Print and shaded views of the part. All mm, measured from the part's lowest x, y and z. A direction names the side the tool comes from. Give positions to 0.01 mm unless a question says otherwise; leave off trailing zeros. Order: outer loops, then holes, each group sorted by start corner. A loop starts at its lowest first (then second) coordinate and runs counter-clockwise, first axis right, second up. Notation, with made-up numbers: (-39, -15) - (-25, -15) arc R30 ccw to (-25, 16) - close; hole circle Ø5 at (25.25, 70). An arc over 180 degrees is marked (long way). Answer in a Markdown table with one row per item.
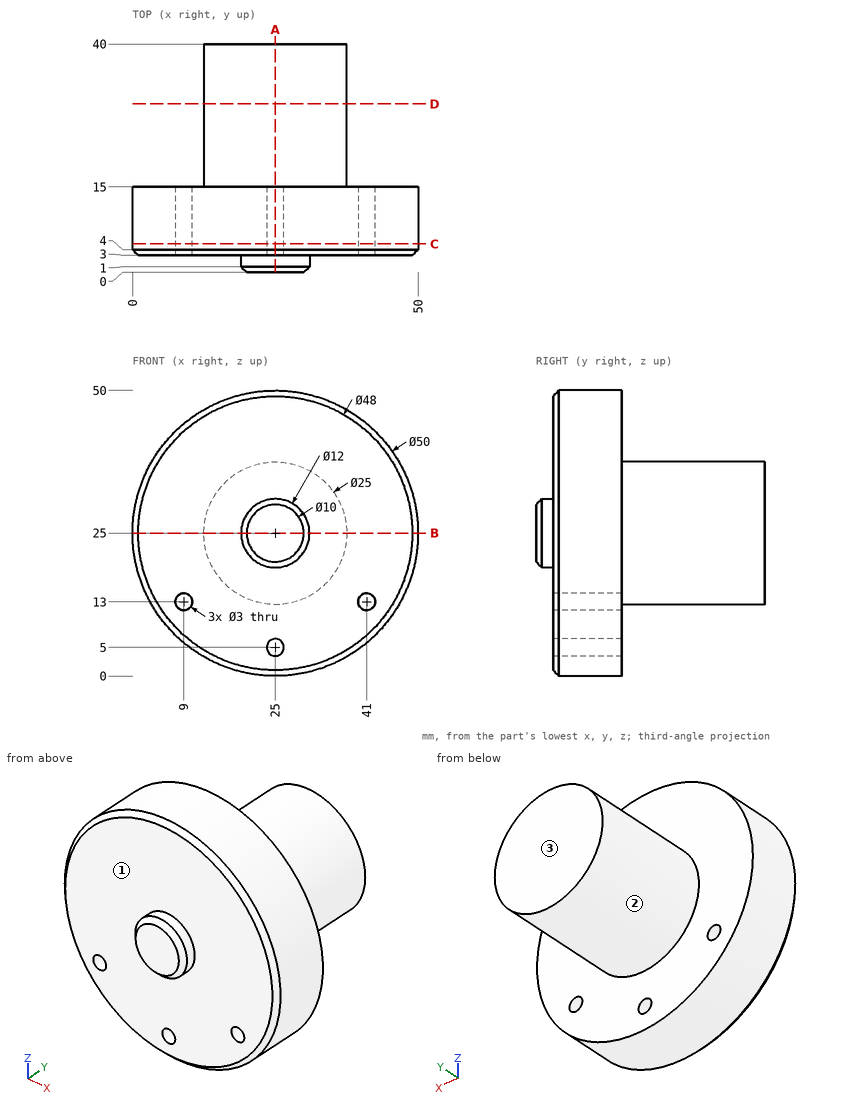
1. Cut at B-B on z = 25. Write the cut outline in (x, y).
Check result:
| item | result |
|---|---|
| outline | (0, 4) - (1, 3) - (19, 3) - (19, 1) - (20, 0) - (30, 0) - (31, 1) - (31, 3) - (49, 3) - (50, 4) - (50, 15) - (37.5, 15) - (37.5, 40) - (12.5, 40) - (12.5, 15) - (0, 15) - close |
2. Cut at D-D on y = 29.5. Write the cut outline in (x, z), and give its area (3 significant figures).
Check result:
| item | result |
|---|---|
| outline | circle Ø25 at (25, 25) |
| area | 491 mm² |
3. Probe line 1 (X direction, y = 9.5, z = 13); line 2 (Y direction, x = 40, z = 16.5); line 3 (Y direction, x = 15, z = 18.5). List the from-to ranges inside material, lowest first.
Check result:
| item | result |
|---|---|
| line 1 | x = 3.07 to 7.5, 10.5 to 39.5, 42.5 to 46.93 |
| line 2 | y = 3 to 15 |
| line 3 | y = 3 to 40 |
4. Cut at C-C on y = 5. Write the cut outline in (x, z), and give its area (3 significant figures).
Check result:
| item | result |
|---|---|
| outline | circle Ø50 at (25, 25); hole circle Ø3 at (9, 13); hole circle Ø3 at (25, 5); hole circle Ø3 at (41, 13) |
| area | 1,940 mm² |
5. Cut at A-A on x = 25. Write the cut outline in (y, z), and give its area (3 significant figures).
Check result:
| item | result |
|---|---|
| outline | (0, 20) - (1, 19) - (3, 19) - (3, 6.5) - (15, 6.5) - (15, 12.5) - (40, 12.5) - (40, 37.5) - (15, 37.5) - (15, 50) - (4, 50) - (3, 49) - (3, 31) - (1, 31) - (0, 30) - close; (3, 1) - (4, 0) - (15, 0) - (15, 3.5) - (3, 3.5) - close |
| area | 1,220 mm² |
6. Which spindle directions (+Z, -Z, +X, -X, +Y, -Y) get a long thin tool onto all of the face, cutting with end or side? Do the marked faces 1, 2 and 3. Say none if no direction does.
Check result:
| item | result |
|---|---|
| face 1 | -Y |
| face 2 | +Y |
| face 3 | +Z, -Z, +X, -X, +Y |
7. Drop flat-ended pins along their axis: P1, Ø5, axis at x = 44.5, z = 13, coming from the -Y side; P2, Ø6, axis at x = 19.5, y = 20.5, coming from the -Z side; P3, Ø1.5, axis at x = 28, z = 31, coming from the -Y side; P4, Ø2.5, axis at x = 41, z = 13, coming from the +Y side. Give the stop position or say it passes through.
Check result:
| item | result |
|---|---|
| P1 | stops at y = 3 |
| P2 | stops at z = 12.75 |
| P3 | stops at y = 0.96 |
| P4 | passes through |
